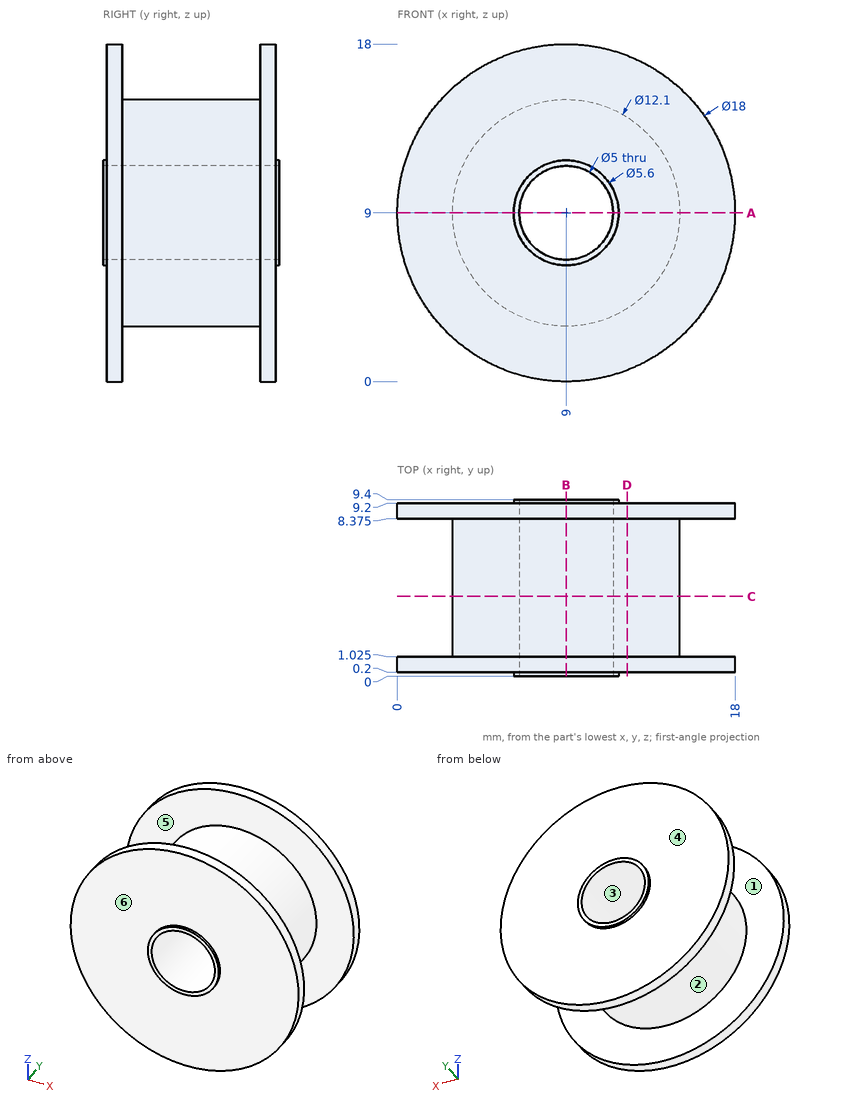
Geometry check sheet. Reference: drawing and pictorial views, mm from the part's lowest x, y, z. A direction names the side the tool comes from. Give positions to 0.01 mm unless a question says otherwise; leave off trailing zeros. Order: outer loops, then holes, each group sorted by start corner. A loop starts at its lowest first (then second) coordinate and runs counter-clockwise, first axis right, second up. Notation, with made-up numbers: M 24.25,37.5 L 76.25,37.5 A16 cw 76.25,43.5 Z; hole C 89,44 d9. An arc over 180 degrees is marked long. Return JSON: item names as keys, results as strings. Group by question number.
1) Access from +Z, -Z, +X, -X, +Y, -Y to the whole of each face (thin tool, end or side, straight path). Record for the marked faces 4, 5 and 6.
2) Section check D-D on x = 12.25. Record the cut outline in (y, z) (3 decimals).
3) Section check C-C on y = 4.25. Record the cut outline in (x, z).
4) Scan lines: line 1 (Y direction, x = 16.25, z = 4.75) (3 decimals); line 2 (X direction, y = 3.25, z = 9); line 3 (Y direction, x = 11.75, z = 10.75). Record each from-to range of solid material in increasing order.
5) Mould release check, pull along Z, two halves, no side actions. Record for the marked faces 1, 2 and 3: pulls with the +Z half, pulls with the -Z half, needs draft (parallel to the pull), parting line crosses it, or undercut.
6) Section check B-B on x = 9. Record the cut outline in (y, z) (3 decimals), and give its area (3 significant figures).
7) Section check A-A on z = 9. Record the cut outline in (x, y) (3 decimals), and give its area (3 significant figures).
8) Go/stop test with flat-tipped pins: pin 1 Ø1 at (x, y) = (5.5, 3.5) entering from +Z; pin 2 Ø1 at (x, z) = (10.5, 15.5) entering from +Y; pin 3 Ø1.5 at (x, y) = (8.5, 2.5) entering from +Z. Record where each tip stops, or that it passes through.
Answer block:
{
 "1": {"face 4": "+Y", "face 5": "none", "face 6": "-Y"},
 "2": {"outline": "M 0.2,0.607 L 1.025,0.607 L 1.025,3.897 L 8.375,3.897 L 8.375,0.607 L 9.2,0.607 L 9.2,17.393 L 8.375,17.393 L 8.375,14.103 L 1.025,14.103 L 1.025,17.393 L 0.2,17.393 Z"},
 "3": {"outline": "C 9,9 d12.1; hole C 9,9 d5"},
 "4": {"line 1": "y = 0.2 to 1.025, 8.375 to 9.2", "line 2": "x = 2.95 to 6.5, 11.5 to 15.05", "line 3": "y = 0.2 to 9.2"},
 "5": {"face 1": "needs draft", "face 2": "parting line crosses it", "face 3": "undercut"},
 "6": {"outline": "M 0,6.2 L 0.2,6.2 L 0.2,0 L 1.025,0 L 1.025,2.95 L 8.375,2.95 L 8.375,0 L 9.2,0 L 9.2,6.2 L 9.4,6.2 L 9.4,6.5 L 0,6.5 Z; M 0,11.5 L 9.4,11.5 L 9.4,11.8 L 9.2,11.8 L 9.2,18 L 8.375,18 L 8.375,15.05 L 1.025,15.05 L 1.025,18 L 0.2,18 L 0.2,11.8 L 0,11.8 Z", "area": "73.9 mm^2"},
 "7": {"outline": "M 0,0.2 L 6.2,0.2 L 6.2,0 L 6.5,0 L 6.5,9.4 L 6.2,9.4 L 6.2,9.2 L 0,9.2 L 0,8.375 L 2.95,8.375 L 2.95,1.025 L 0,1.025 Z; M 11.5,0 L 11.8,0 L 11.8,0.2 L 18,0.2 L 18,1.025 L 15.05,1.025 L 15.05,8.375 L 18,8.375 L 18,9.2 L 11.8,9.2 L 11.8,9.4 L 11.5,9.4 Z", "area": "73.9 mm^2"},
 "8": {"pin 1": "stops at z = 14.25", "pin 2": "stops at y = 9.2", "pin 3": "stops at z = 15.05"}
}
